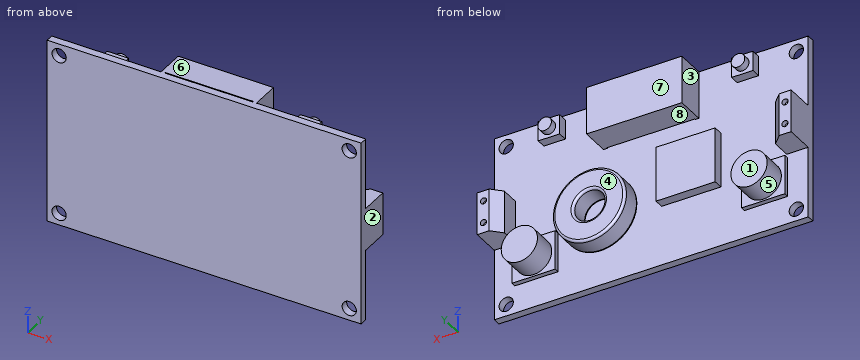
from build123d import *

# Parameters (mm, degrees)
SKETCH_1_W          = 66
SKETCH_1_H          = 39
EXTRUDE_1_DEPTH     = 1.6
SKETCH_2_R          = 1.5
CUT_EXTRUDE_1_DEPTH = 1.6
SKETCH_3_W          = 4.5
SKETCH_3_H          = 9
EXTRUDE_2_DEPTH     = 6
CHAMFER_1_SIZE      = 2
SKETCH_6_R          = 0.65
CUT_EXTRUDE_2_DEPTH = 1
SKETCH_7_W          = 20.048070128
SKETCH_7_H          = 10.01913925
EXTRUDE_3_DEPTH     = 6
SKETCH_8_W          = 18.487369842
SKETCH_8_H          = 0.2
CUT_EXTRUDE_3_DEPTH = 45.571855355
SKETCH_9_R          = 7.645962027
SKETCH_9_R_2        = 3.237215686
EXTRUDE_4_DEPTH     = 4.5
FILLET_1_R          = 0.5
SKETCH_10_W         = 9.085824886
SKETCH_10_H         = 8.295753157
SKETCH_10_R         = 3.812502592
EXTRUDE_5_DEPTH     = 1
SKETCH_11_R         = 3.812502592
EXTRUDE_6_DEPTH     = 5
SKETCH_12_W         = 12.443629735
SKETCH_12_H         = 11.614054419
EXTRUDE_7_DEPTH     = 2
SKETCH_13_W         = 4.503408857
SKETCH_13_H         = 4.147876578
EXTRUDE_8_DEPTH     = 2
SKETCH_14_R         = 1.427058518
EXTRUDE_9_DEPTH     = 1.5


with BuildPart() as part:
    # 草图1 → 凸台-拉伸1 (new body)
    with BuildSketch(Plane(origin=(0, 0, 0), x_dir=(1, 0, 0), z_dir=(0, 1, 0))):
        Rectangle(SKETCH_1_W, SKETCH_1_H)
    extrude(amount=EXTRUDE_1_DEPTH)

    # 草图2 → 切除-拉伸1 (cut)
    with BuildSketch(Plane(origin=(0, 1.6, 0), x_dir=(1, 0, 0), z_dir=(0, 1, 0))):
        with Locations(Location((-30.5, -17, 0), (0, 0, 270))):
            Circle(SKETCH_2_R)
        with Locations(Location((30.5, -17, 0), (0, 0, 90))):
            Circle(SKETCH_2_R)
        with Locations(Location((30.5, 17, 0), (0, 0, 270))):
            Circle(SKETCH_2_R)
        with Locations(Location((-30.5, 17, 0), (0, 0, 90))):
            Circle(SKETCH_2_R)
    extrude(amount=-CUT_EXTRUDE_1_DEPTH, mode=Mode.SUBTRACT)

    # 草图3 → 凸台-拉伸2 (add)
    with BuildSketch(Plane(origin=(0, 1.6, 0), x_dir=(1, 0, 0), z_dir=(0, 1, 0))):
        with Locations((-30.75, 0)):
            Rectangle(SKETCH_3_W, SKETCH_3_H)
        with Locations((30.75, 0)):
            Rectangle(SKETCH_3_W, SKETCH_3_H)
    extrude(amount=EXTRUDE_2_DEPTH)

    # 倒角1
    chamfer_1_edges = [part.edges().sort_by_distance(p)[0] for p in [
        (-28.5, 7.6, 0),
        (28.5, 7.6, 0),
    ]]
    chamfer(chamfer_1_edges, length=CHAMFER_1_SIZE)

    # 草图6 → 切除-拉伸2 (cut)
    with BuildSketch(Plane(origin=(0, 7.6, 0), x_dir=(1, 0, 0), z_dir=(0, 1, 0))):
        with Locations(Location((-31.719459614, 2.331808923, 0), (0, 0, 270))):
            Circle(SKETCH_6_R)
        with Locations(Location((-31.719459614, -2.331808923, 0), (0, 0, 270))):
            Circle(SKETCH_6_R)
        with Locations(Location((31.687681101, -2.331808923, 0), (0, 0, 270))):
            Circle(SKETCH_6_R)
        with Locations(Location((31.687681101, 2.331808923, 0), (0, 0, 270))):
            Circle(SKETCH_6_R)
    extrude(amount=-CUT_EXTRUDE_2_DEPTH, mode=Mode.SUBTRACT)

    # 草图7 → 凸台-拉伸3 (add)
    with BuildSketch(Plane(origin=(0, 1.6, 0), x_dir=(1, 0, 0), z_dir=(0, 1, 0))):
        with Locations((0, -14.490430375)):
            Rectangle(SKETCH_7_W, SKETCH_7_H)
    extrude(amount=EXTRUDE_3_DEPTH)

    # 草图8 → 切除-拉伸3 (cut, through all)
    with BuildSketch(Plane(origin=(0, 0, 9.48086075), x_dir=(-1, 0, 0), z_dir=(0, 0, -1))):
        with Locations((0, 1.7)):
            Rectangle(SKETCH_8_W, SKETCH_8_H)
    extrude(amount=-CUT_EXTRUDE_3_DEPTH, mode=Mode.SUBTRACT)


with BuildPart() as body_2:
    # 草图9 → 凸台-拉伸4 (new body)
    with BuildSketch(Plane(origin=(0, 1.6, 0), x_dir=(1, 0, 0), z_dir=(0, 1, 0))):
        with Locations(Location((10.458848846, 4.732200461, 0), (0, 0, 270))):
            Circle(SKETCH_9_R)
        with Locations(Location((10.458848846, 4.732200461, 0), (0, 0, 270))):
            Circle(SKETCH_9_R_2, mode=Mode.SUBTRACT)
    extrude(amount=EXTRUDE_4_DEPTH)

    # 圆角1
    fillet_1_edges = [body_2.edges().sort_by_distance(p)[0] for p in [
        (10.458848846, 1.6, -12.378162489),
        (10.458848846, 6.1, -12.378162489),
        (10.458848846, 1.6, -7.969416147),
        (10.458848846, 6.1, -7.969416147),
    ]]
    fillet(fillet_1_edges, radius=FILLET_1_R)


with BuildPart() as part_1:
    add(part.part)

    # 相交1: read off the stored shape, not the designer's step
    # 相交1: union body 2
    add(body_2.part)

    # 草图10 → 凸台-拉伸5 (add)
    # profile 1 of 3: a face of its own
    with BuildSketch(Plane(origin=(0, 1.6, 0), x_dir=(1, 0, 0), z_dir=(0, 1, 0))):
        with Locations((24.146567223, 9.480860751)):
            Rectangle(SKETCH_10_W, SKETCH_10_H)
        with Locations((24.146567223, 9.48086075)):
            Circle(SKETCH_10_R, mode=Mode.SUBTRACT)
    # profile 2 of 3: a face of its own
    with BuildSketch(Plane(origin=(0, 1.6, 0), x_dir=(1, 0, 0), z_dir=(0, 1, 0))):
        with Locations((24.146567223, 9.48086075)):
            Circle(SKETCH_10_R)
    # profile 3 of 3: a face of its own
    with BuildSketch(Plane(origin=(0, 1.6, 0), x_dir=(1, 0, 0), z_dir=(0, 1, 0))):
        with Locations((-24.146567223, 9.480860751)):
            Rectangle(SKETCH_10_W, SKETCH_10_H)
    extrude(amount=EXTRUDE_5_DEPTH)

    # 草图11 → 凸台-拉伸6 (add)
    with BuildSketch(Plane(origin=(0, 2.6, 0), x_dir=(1, 0, 0), z_dir=(0, 1, 0))):
        with Locations(Location((-24.146567223, 9.48086075, 0), (0, 0, 270))):
            Circle(SKETCH_11_R)
        with Locations(Location((24.146567223, 9.48086075, 0), (0, 0, 270))):
            Circle(SKETCH_11_R)
    extrude(amount=EXTRUDE_6_DEPTH)

    # 草图12 → 凸台-拉伸7 (add)
    with BuildSketch(Plane(origin=(0, 1.6, 0), x_dir=(1, 0, 0), z_dir=(0, 1, 0))):
        with Locations((-8.414263916, 1.066596835)):
            Rectangle(SKETCH_12_W, SKETCH_12_H)
    extrude(amount=EXTRUDE_7_DEPTH)

    # 草图13 → 凸台-拉伸8 (add)
    with BuildSketch(Plane(origin=(0, 1.6, 0), x_dir=(1, 0, 0), z_dir=(0, 1, 0))):
        with Locations((-20.324595233, -16.532250933)):
            Rectangle(SKETCH_13_W, SKETCH_13_H)
        with Locations((20.324595233, -16.532250933)):
            Rectangle(SKETCH_13_W, SKETCH_13_H)
    extrude(amount=EXTRUDE_8_DEPTH)

    # 草图14 → 凸台-拉伸9 (add)
    with BuildSketch(Plane(origin=(0, 3.6, 0), x_dir=(1, 0, 0), z_dir=(0, 1, 0))):
        with Locations(Location((-20.324595233, -16.532250933, 0), (0, 0, 270))):
            Circle(SKETCH_14_R)
        with Locations(Location((20.324595233, -16.532250933, 0), (0, 0, 270))):
            Circle(SKETCH_14_R)
    extrude(amount=EXTRUDE_9_DEPTH)


solid = part_1.part
Source: CAD feature listing. Evaluate the final solid. Frame: model axes, mm. Face numbers are marked on the shaded views. A direction names the side the tool comes from. Give positions to 0.01 mm unless a question says otherwise; leave off trailing zeros. Write each loop counter-clockwise with the first axis right and the second up, starting at its lowest first coordinate (ties: lowest second). Pieces come first, ordered by that corner, then holes. Notation, with made-up numbers: (-31, 2) - (24, 2) arc R20 cw to (24, 9) - close; hole circle Ø4 at (59.5, 49). An arc over 180 degrees is marked (long way). Write item = value, one per line. Start each with the question number.
Q1. Pin query (flat end, axial travel): pin 1 Ø0.6 at (y, z) = (3, 17.5) entering from +X; pin 2 Ø3 at (x, z) = (0, -4.5) entering from +Y; pin 3 Ø3.5 at (x, z) = (-19.5, 16.5) entering from +Y. Return the tip coordinate at first contact, or that it passes through.
Q2. Draft query along Z for the marked faces 6, 7 and 8. Return one class per face: +Z half, -Z half, draft (parallel to the pull), parting line (faces both ways), or undercut.
Q3. Cut plane C-C, the plane x = -17. Return loops of the section in (y, z), then the cut area to 3 significant figures.
Q4. Reachability of the marked faces 1, 2, 3, 4 and 5 from +Z, -Z, +X, -X, +Y, -Y: full face, straight path, thin tool, end or side. Return the list, or none.
Q5. Cut plane B-B, the plane z = 17. Give the number of separate pieces and of enclosed holes in the cut face, then the cut area to 3 significant figures.
Q6. Material intervals for probe 1 along Z at (x, y) = (30, 0.5); probe 2 along Z at (x, y) = (-3, 2); probe 3 along X at (y, z) = (0.9, 17), sorted ascending.
Q7. Cut plane A-A, the plane z = 6.5. Return loops of the section in (x, y), then the cut area to 3 significant figures.
Computed values:
q1.pin_1 = 22.58
q1.pin_2 = 1.6
q1.pin_3 = 5.1
q2.face_6 = +Z half
q2.face_7 = draft
q2.face_8 = undercut
q3.outline = (0, -19.5) - (1.6, -19.5) - (1.6, 19.5) - (0, 19.5) - close
q3.area = 62.4 mm²
q4.face_1 = +Z, -Z, +X, -X, +Y
q4.face_2 = +Z, -Z, +X, +Y, -Y
q4.face_3 = +Z, +Y
q4.face_4 = -Z, +Y
q4.face_5 = +Y
q5.separate_pieces = 3
q5.enclosed_holes = 1
q5.area = 239 mm²
q6.probe_1 = -19.5 to -18.41, -15.59 to 15.59, 18.41 to 19.5
q6.probe_2 = -6.87 to 4.74, 9.48 to 19.5
q6.probe_3 = -33 to -32, -29 to 29, 32 to 33
q7.outline = (-33, 0) - (33, 0) - (33, 1.6) - (-33, 1.6) - close
q7.area = 106 mm²
